from build123d import *

# Parameters (mm, degrees)
BOSS_EXTRU_7_DEPTH         = 5
BOSS_EXTRU_8_DEPTH         = 12
ESQUISSE25_R               = 9.525
ENL_V_MAT_EXTRU_1_DEPTH    = 10
R_P_TITION_LIN_AIRE2_COUNT = 2
R_P_TITION_LIN_AIRE2_PITCH = 30
ESQUISSE22_R               = 4.1
BOSS_EXTRU_9_DEPTH         = 5
ESQUISSE26_R               = 6.5
ENL_V_MAT_EXTRU_2_DEPTH    = 163.491730559
BOSS_EXTRU_10_START        = -90
BOSS_EXTRU_10_DEPTH        = 78


with BuildPart() as part:
    # Esquisse20 → Boss.-Extru.7 (new body)
    with BuildSketch(Plane.XZ):
        Polygon((-25, 0), (-15, 17.320508076), (-15, 90), (15, 90), (15, 17.320508076), (25, 0), align=None)
    extrude(amount=-BOSS_EXTRU_7_DEPTH)

    # Esquisse21 → Boss.-Extru.8 (add)
    with BuildSketch(Plane.XY.offset(90)):
        with BuildLine():
            Line((-15, 5), (-11, 9.76701437))
            Line((-11, 9.76701437), (-11, 26.15))
            ThreePointArc((-11, 26.15), (0, 37.15), (11, 26.15))
            Line((11, 26.15), (11, 9.76701437))
            Line((11, 9.76701437), (15, 5))
            Line((15, 5), (-15, 5))
        make_face()
    boss_extru_8 = extrude(amount=-BOSS_EXTRU_8_DEPTH)

    # Esquisse25 → Enlèv. mat.-Extru.1 (cut)
    with BuildSketch(Plane.XY.offset(90)):
        with Locations((0, 26.15)):
            Circle(ESQUISSE25_R)
    enl_v_mat_extru_1 = extrude(amount=-ENL_V_MAT_EXTRU_1_DEPTH, mode=Mode.SUBTRACT)

    # Répétition linéaire2: Boss.-Extru.8, Enlèv. mat.-Extru.1 ×2
    with Locations(*[(0, 0, -i * R_P_TITION_LIN_AIRE2_PITCH) for i in range(1, R_P_TITION_LIN_AIRE2_COUNT)]):
        add(boss_extru_8)
        add(enl_v_mat_extru_1, mode=Mode.SUBTRACT)

    # Esquisse22 → Boss.-Extru.9 (add)
    with BuildSketch(Plane(origin=(0, 5, 0), x_dir=(1, 0, 0), z_dir=(0, 1, 0))):
        Polygon((-25, 0), (25, 0), (25, 38.1), (25, 76.2), (-25, 76.2), (-25, 38.1), align=None)
        with Locations(Location((-15, 19.05, 0), (0, 0, 270))):
            Circle(ESQUISSE22_R, mode=Mode.SUBTRACT)
        with Locations(Location((15, 19.05, 0), (0, 0, 270))):
            Circle(ESQUISSE22_R, mode=Mode.SUBTRACT)
        with Locations(Location((19.05, 56.934132562, 0), (0, 0, 270))):
            Circle(ESQUISSE22_R, mode=Mode.SUBTRACT)
        with Locations(Location((-19.05, 56.934132562, 0), (0, 0, 270))):
            Circle(ESQUISSE22_R, mode=Mode.SUBTRACT)
    extrude(amount=-BOSS_EXTRU_9_DEPTH)

    # Esquisse26 → Enlèv. mat.-Extru.2 (cut, through all)
    with BuildSketch(Plane.XY.offset(80)):
        with Locations((0, 26.15)):
            Circle(ESQUISSE26_R)
    extrude(amount=-ENL_V_MAT_EXTRU_2_DEPTH, mode=Mode.SUBTRACT)

    # Esquisse27 → Boss.-Extru.10 (add)
    with BuildSketch(Plane.XY.offset(90).offset(BOSS_EXTRU_10_START)):
        Polygon((-11, 9.76701437), (-11, 5), (-15, 5), align=None)
        Polygon((15, 5), (11, 9.76701437), (11, 5), align=None)
    extrude(amount=BOSS_EXTRU_10_DEPTH)


solid = part.part
For this review, take the finished solid that the model builds, in its own axes (mm). A direction names the side the tool comes from. Give positions to 0.01 mm unless a question says otherwise; leave off trailing zeros. Loops run counter-clockwise (first coordinate to the right, second up) from the corner with the lowest first, then second, coordinate; pieces in that order, holes last. Notation, with made-up numbers: (87.25, 6.5) - (101.25, 6.5) arc R21 ccw to (101.25, 20.5) - close; hole circle Ø4 at (61.5, -1). An arc over 180 degrees is marked (long way). Write each question's results on one line, items separated by ' | '.
(1) Take a section at C-C (y = 30.5). Give the boundary of the cut face in (x, z), then the cut area to 3 significant figures.
Conclusion:
outline: (-10.1, 48) - (-4.83, 48) - (-4.83, 50) - (-8.47, 50) - (-8.47, 60) - (-10.1, 60) - close; (-10.1, 78) - (-4.83, 78) - (-4.83, 80) - (-8.47, 80) - (-8.47, 90) - (-10.1, 90) - close; (4.83, 48) - (10.1, 48) - (10.1, 60) - (8.47, 60) - (8.47, 50) - (4.83, 50) - close; (4.83, 78) - (10.1, 78) - (10.1, 90) - (8.47, 90) - (8.47, 80) - (4.83, 80) - close | area: 107 mm^2
(2) For line 1 along X through (y, z) = (2, -19); line 2 along Y through (x, z) = (0, 49); line 3 along Y through (x, z) = (-13, -3), list the stretches that pass through material, from the lowest coordinate up.
Conclusion:
line 1: -25 to -19.1, -10.9 to 10.9, 19.1 to 25 | line 2: 0 to 19.65, 32.65 to 37.15 | line 3: 0 to 5
(3) Take a section at A-A (y = 12). Give the boundary of the cut face in (x, z).
Conclusion:
outline: (-11, 48) - (11, 48) - (11, 60) - (-11, 60) - close; (-11, 78) - (11, 78) - (11, 90) - (-11, 90) - close
(4) Take a section at D-D (z = 27). Give the boundary of the cut face in (x, y).
Conclusion:
outline: (-15, 0) - (15, 0) - (15, 5) - (11, 9.77) - (11, 5) - (-11, 5) - (-11, 9.77) - (-15, 5) - close
(5) Take a section at B-B (x = 0). Give the boundary of the cut face in (y, z) (3 decimals), then the cut area to 3 significant figures.
Conclusion:
outline: (0, -76.2) - (5, -76.2) - (5, 48) - (19.65, 48) - (19.65, 50) - (16.625, 50) - (16.625, 60) - (5, 60) - (5, 78) - (19.65, 78) - (19.65, 80) - (16.625, 80) - (16.625, 90) - (0, 90) - close; (32.65, 48) - (37.15, 48) - (37.15, 60) - (35.675, 60) - (35.675, 50) - (32.65, 50) - close; (32.65, 78) - (37.15, 78) - (37.15, 90) - (35.675, 90) - (35.675, 80) - (32.65, 80) - close | area: 1,170 mm^2
(6) Draft analysis for pull direction Y (two halves, no side actions). For faces 1 (the flat face through (-13.03, 7.35, 44.37)), 2 (the flat face through (-2.3, 19.9, 80)), 3 (the flat face through (0, 3, -76.2)), state which applies: +Y half, -Y half, draft (parallel to the pull), parting line (faces both ways), or undercut.
Conclusion:
face 1: +Y half | face 2: undercut | face 3: draft
(7) For pin 1 Ø15 at (x, y) = (0, 26.15) entering from -Z; pin 2 Ø1.5 at (y, z) = (3, 56.5) entering from +X; pin 3 Ø6 at (x, z) = (14, -44) entering from +Y, all flat-tipped, find the tip position at first contact; note any pin that passes through.
Conclusion:
pin 1: z = 48 | pin 2: x = 15 | pin 3: y = 5
(8) For faces 4 (the flat face through (0, 14, 60)), 5 (the flat face through (-15, 2, 53)), 6 (the flat face through (-12, 6, 0)), 7 (the flat face through (-11, 18, 84)), list the 3-axis set-ups (+Z, -Z, +X, -X, +Y, -Y) from which the entire face can be reached by the end or side of a thin tool; tool diameter is ignored.
Conclusion:
face 4: +Y | face 5: +Z, -X, +Y, -Y | face 6: -Z, +X, -X, +Y | face 7: +Z, -Z, -X, +Y
